The figure shows three views and two pictorial views of one solid part (mm, origin at its lowest corner). Answer the questions. A direction names the side the tool comes from. Round coordinates to 2 decimals unless told otherwise and drop trailing zeros. Order: outer loops, then holes, each group sorted by start corner. A loop starts at its lowest first (then second) coordinate and runs counter-clockwise, first axis right, second up. Notation, with made-up numbers: (-34.75, 14) -> (9.25, 14) arc R25 cw to (9.25, 26) -> close; hole circle Ø5 at (40, 50). An arc over 180 degrees is marked (long way). One line per item, written item: value. Start each with the question number.
1. Consider line 1 (Y direction, x = 150.5, z = 28.5) (1 decimal); line 2 (Z direction, x = 37.5, y = 21.25). Determine where each line is inside the solid, lowest interval first.
2. Section D-D (x = 219) is taken. Give the vertices of the cut face in (y, z) (1 decimal), then the cut area to 3 significant figures.
3. Section A-A (x = 12.7) is taken. Give the vertices of the cut face in (y, z) (1 decimal).
4. Section C-C (z = 3.5) is taken. Give the vertices of the cut face in (x, y) (1 decimal).
5. For the marked faces 1 and 2, determine the directions among +Z, -Z, +X, -X, +Y, -Y from which every point of the face is accessible in a straight line to the end or side of a thin tool.
6. Section B-B (y = 21.5) is taken. Give the vertices of the cut face in (x, z).
7. Flat-ended cylindrical pins translate along their axes: pin 1 Ø4 at (x, y) = (192, 8.5) entering from -Z; pin 2 Ø1.5 at (x, z) = (245.5, 26) entering from +Y (3 decimals). Find the tip coordinate at first contact, or state that the pin passes through.
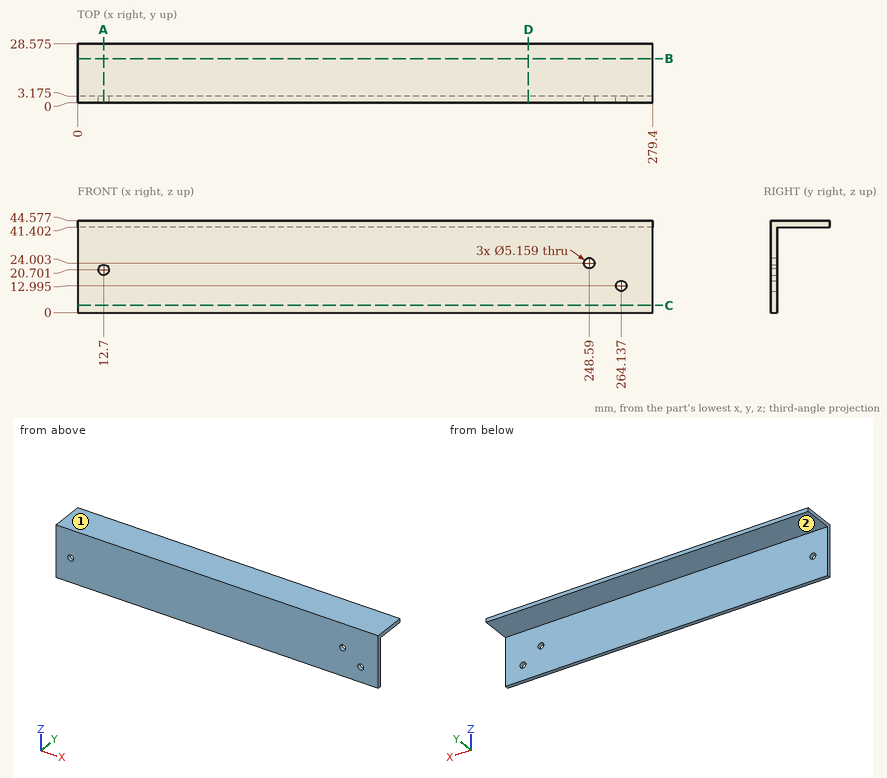
Answer:
1. line 1: 0 to 3.2
1. line 2: 41.4 to 44.58
2. outline: (0, 0) -> (3.2, 0) -> (3.2, 41.4) -> (28.6, 41.4) -> (28.6, 44.6) -> (0, 44.6) -> close
2. area: 222 mm^2
3. outline: (0, 0) -> (3.2, 0) -> (3.2, 18.1) -> (0, 18.1) -> close; (0, 23.3) -> (3.2, 23.3) -> (3.2, 41.4) -> (28.6, 41.4) -> (28.6, 44.6) -> (0, 44.6) -> close
4. outline: (0, 0) -> (279.4, 0) -> (279.4, 3.2) -> (0, 3.2) -> close
5. face 1: +Z, +X, -X, +Y, -Y
5. face 2: -Z, +X, -X, +Y
6. outline: (0, 41.4) -> (279.4, 41.4) -> (279.4, 44.58) -> (0, 44.58) -> close
7. pin 1: z = 41.4
7. pin 2: y = 3.175
